```python
from build123d import *

# Parameters (mm, degrees)
BOSS_EXTRUDE1_DEPTH = 4.3


with BuildPart() as part:
    # Sketch1 → Boss-Extrude1 (new body)
    with BuildSketch(Plane.XY):
        Polygon((-8, 2.65), (-8, 20), (8, 20), (8, 2.65), (12.3, 2.65), (12.3, -12.65), (8, -12.65), (8, -20), (-8, -20), (-8, -12.65), (-12.3, -12.65), (-12.3, 2.65), align=None)
        with BuildLine():
            Line((-1.5, -16), (-1.5, 16))
            ThreePointArc((-1.5, 16), (0, 17.5), (1.5, 16))
            Line((1.5, 16), (1.5, -16))
            ThreePointArc((1.5, -16), (0, -17.5), (-1.5, -16))
        make_face(mode=Mode.SUBTRACT)
    extrude(amount=BOSS_EXTRUDE1_DEPTH)


solid = part.part
```
Can you work these out from the model? Positions are in its coordinate system, mm. A direction names the side the tool comes from. Round coordinates to 2 decimals unless told otherwise and drop trailing zeros. Loops run counter-clockwise (first coordinate to the right, second up) from the corner with the lowest first, then second, coordinate; pieces in that order, holes last. Notation, with made-up numbers: (-29, -12) -> (12, -12) arc R33 ccw to (12, 25) -> close; hole circle Ø5 at (39.25, 77.5). An arc over 180 degrees is marked (long way). Answer in a Markdown table with one row per item.
Item 1: Suppose I cut it at A-A, the plane y = 6. List the corners of the cut face in (x, z) for me, plus the area to 3 significant figures.
Answer block:
| item | result |
|---|---|
| outline | (-8, 0) -> (-1.5, 0) -> (-1.5, 4.3) -> (-8, 4.3) -> close; (1.5, 0) -> (8, 0) -> (8, 4.3) -> (1.5, 4.3) -> close |
| area | 55.9 mm² |
Item 2: Will these pins go through, and if not, where does the flat tip stop? P1, Ø2, axis at y = 8.5, z = 3, coming from the +X side; P2, Ø2, axis at x = -10, z = 3, coming from the -Y side; P3, Ø2, axis at x = -6, y = 3, coming from the -Z side.
Answer block:
| item | result |
|---|---|
| P1 | x = 8 |
| P2 | y = -12.65 |
| P3 | z = 0 |
Item 3: On a 3-axis mill with a long thin cutter (end or side, diameter ignored), from which of +Z, -Z, +X, -X, +Y, -Y can I reach the whole of each face in a straight line? I mean faces 4 (the flat face through (-10, 2.65, 2)), 5 (the flat face through (8, -16, 2)), 6 (the flat face through (8, 11, 2)), 7 (the flat face through (-8, -16, 2)), 8 (the cylindrical face through (0, -17.5, 2.1)). Say none if no direction works.
Answer block:
| item | result |
|---|---|
| face 4 | +Z, -Z, -X, +Y |
| face 5 | +Z, -Z, +X, -Y |
| face 6 | +Z, -Z, +X, +Y |
| face 7 | +Z, -Z, -X, -Y |
| face 8 | +Z, -Z |
Item 4: Suppose I cut it at B-B, the plane z = 3.5. List the corners of the cut face in (x, y) for me.
Answer block:
| item | result |
|---|---|
| outline | (-12.3, -12.65) -> (-8, -12.65) -> (-8, -20) -> (8, -20) -> (8, -12.65) -> (12.3, -12.65) -> (12.3, 2.65) -> (8, 2.65) -> (8, 20) -> (-8, 20) -> (-8, 2.65) -> (-12.3, 2.65) -> close; hole (-1.5, -16) arc R1.5 ccw to (1.5, -16) -> (1.5, 16) arc R1.5 ccw to (-1.5, 16) -> close |
Item 5: Suppose I cut it at C-C, the plane x = 0. List the corners of the cut face in (y, z) for me, plus the area to 3 significant figures.
Answer block:
| item | result |
|---|---|
| outline | (-20, 0) -> (-17.5, 0) -> (-17.5, 4.3) -> (-20, 4.3) -> close; (17.5, 0) -> (20, 0) -> (20, 4.3) -> (17.5, 4.3) -> close |
| area | 21.5 mm² |
Item 6: If I drill on probe 1 along X at (y, z) = (-1, 3.4); probe 2 along X at (y, z) = (-13.5, 3.2); probe 3 along Y at (x, z) = (0, 1.2), over which ranges is the centre line in solid material (lowest first)?
Answer block:
| item | result |
|---|---|
| probe 1 | -12.3 to -1.5, 1.5 to 12.3 |
| probe 2 | -8 to -1.5, 1.5 to 8 |
| probe 3 | -20 to -17.5, 17.5 to 20 |
Item 7: Suppose I cut it at D-D, the plane y = -18. List the corners of the cut face in (x, z) for me, plus the area to 3 significant figures.
Answer block:
| item | result |
|---|---|
| outline | (-8, 0) -> (8, 0) -> (8, 4.3) -> (-8, 4.3) -> close |
| area | 68.8 mm² |
Item 8: We'd pull the mould along Y, two halves only. Please class faces 1 (the flat face through (0, 20, 2)), 2 (the flat face through (1.5, 0, 2)), 3 (the flat face through (-10, -12.65, 2)): released by +Y, released by -Y, zero draft, split by the parting line, or undercut.
Answer block:
| item | result |
|---|---|
| face 1 | released by +Y |
| face 2 | undercut |
| face 3 | released by -Y |
